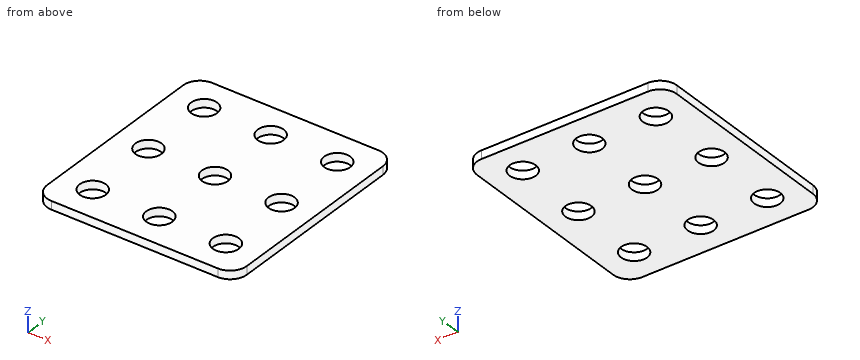
from build123d import *

# Parameters (mm, degrees)
SKETCH1_W           = 38.1
SKETCH1_H           = 41.275
SKETCH1_R           = 2.4892
BOSS_EXTRUDE1_DEPTH = 0.79375
LPATTERN1_START     = -0.79375
LPATTERN1_OUTLINE_R = 2.4892
LPATTERN1_DEPTH     = 1.5875
FILLET1_R           = 3.175


# Read off the part's stored shape, not the designer's step: LPattern1
with BuildPart() as part:
    # Sketch1 → Boss-Extrude1 (new, symmetric)
    with BuildSketch(Plane.XY):
        with Locations((19.05, 20.6375)):
            Rectangle(SKETCH1_W, SKETCH1_H)
        with Locations((6.35, 6.35)):
            Circle(SKETCH1_R, mode=Mode.SUBTRACT)
    extrude(amount=BOSS_EXTRUDE1_DEPTH, both=True)

    # LPattern1 outline → LPattern1 (cut)
    with BuildSketch(Plane.XY.offset(LPATTERN1_START)):
        with Locations((31.75, 34.925)):
            Circle(LPATTERN1_OUTLINE_R)
        with Locations((31.75, 20.6375)):
            Circle(LPATTERN1_OUTLINE_R)
        with Locations((31.75, 6.35)):
            Circle(LPATTERN1_OUTLINE_R)
        with Locations((19.05, 34.925)):
            Circle(LPATTERN1_OUTLINE_R)
        with Locations((19.05, 20.6375)):
            Circle(LPATTERN1_OUTLINE_R)
        with Locations((19.05, 6.35)):
            Circle(LPATTERN1_OUTLINE_R)
        with Locations((6.35, 34.925)):
            Circle(LPATTERN1_OUTLINE_R)
        with Locations((6.35, 20.6375)):
            Circle(LPATTERN1_OUTLINE_R)
    extrude(amount=LPATTERN1_DEPTH, mode=Mode.SUBTRACT)

    # Fillet1
    fillet1_edges = [part.edges().sort_by_distance(p)[0] for p in [
        (0, 41.275, 0),
        (38.1, 41.275, 0),
        (38.1, 0, 0),
        (0, 0, 0),
    ]]
    fillet(fillet1_edges, radius=FILLET1_R)


solid = part.part
Part model, mm, in its own coordinate system. Coordinates: 2 decimals unless noted, no trailing zeros. Write each loop counter-clockwise with the first axis right and the second up, starting at its lowest first coordinate (ties: lowest second). Pieces come first, ordered by that corner, then holes. Notation, with made-up numbers: M 57,-14.5 L 63,-14.5 A32 cw 63,20.5 Z; hole C -27,-29 d2. An arc over 180 degrees is marked long. Return JSON: item names as keys, results as strings.
1. Probe L1, parallel to Y at x = 6.35, z = 0.4 (3 decimals); L2, parallel to X at y = 20.5, z = -0.3; L3, parallel to Y at x = 34, z = 0.2 (3 decimals). List the from-to ranges inside material, lowest first.
Determined:
{"L1": "0 to 3.861, 8.839 to 18.148, 23.127 to 32.436, 37.414 to 41.275", "L2": "0 to 3.86, 8.84 to 16.56, 21.54 to 29.26, 34.24 to 38.1", "L3": "0 to 5.285, 7.415 to 19.573, 21.702 to 33.86, 35.99 to 41.275"}
2. Saw through at C-C, the plane z = -0.3. Count the separate pieces of the cut face and the enclosed holes in it, then the cut area to 3 significant figures.
Determined:
{"separate pieces": "1", "enclosed holes": "9", "area": "1,390 mm²"}
3. Saw through at A-A, the plane x = 6.35. Write the cut outline in (y, z) (3 decimals), then the cut area to 3 significant figures.
Determined:
{"outline": "M 0,-0.794 L 3.861,-0.794 L 3.861,0.794 L 0,0.794 Z; M 8.839,-0.794 L 18.148,-0.794 L 18.148,0.794 L 8.839,0.794 Z; M 23.127,-0.794 L 32.436,-0.794 L 32.436,0.794 L 23.127,0.794 Z; M 37.414,-0.794 L 41.275,-0.794 L 41.275,0.794 L 37.414,0.794 Z", "area": "41.8 mm²"}
4. Flat gauge pin, fed straight in: pin 1 Ø8 at (x, y) = (6.35, 34.925) entering from -Z. Where does the tip first touch, or does it go through?
Determined:
{"pin 1": "z = -0.79"}
5. Saw through at B-B, the plane y = 6.35. Write the cut outline in (x, z).
Determined:
{"outline": "M 0,-0.79 L 3.86,-0.79 L 3.86,0.79 L 0,0.79 Z; M 8.84,-0.79 L 16.56,-0.79 L 16.56,0.79 L 8.84,0.79 Z; M 21.54,-0.79 L 29.26,-0.79 L 29.26,0.79 L 21.54,0.79 Z; M 34.24,-0.79 L 38.1,-0.79 L 38.1,0.79 L 34.24,0.79 Z"}
